Design review of the part built by this model. Coordinates are the model's own, in mm. A direction names the side the tool comes from. Round coordinates to 2 decimals unless told otherwise and drop trailing zeros. Order: outer loops, then holes, each group sorted by start corner. A loop starts at its lowest first (then second) coordinate and runs counter-clockwise, first axis right, second up.
Autodesk Inventor part; units mm, degrees
ref_plane "YZ Plane" through (0, 0, 0) normal (1, 0, 0) x (0, 1, 0)
ref_plane "XZ Plane" through (0, 0, 0) normal (0, 1, 0) x (-1, 0, 0)
ref_plane "XY Plane" through (0, 0, 0) normal (0, 0, 1) x (1, 0, 0)
sketch "Sketch1" plane through (0, 0, 0) normal (0, 1, 0) x (-1, 0, 0)
  line L0 (41.5, -27) -> (-41.5, -27)
  line L1 (-41.5, -27) -> (-41.5, 27)
  line L2 (-41.5, 27) -> (41.5, 27)
  line L3 (41.5, 27) -> (41.5, -27)
  line L4 (41.5, -27) -> (-41.5, 27) construction
  line L5 (-41.5, -27) -> (41.5, 27) construction
  point P0 (0, 0)
  dimension "d0" = 83
  dimension "d1" = 54
extrude "Extrusion1" add sketch "Sketch1" along normal blind 9
sketch "Sketch2" plane through (41.5, 0, 27) normal (1, 0, 0) x (0, 0, -1)
  line L0 (27, 0) -> (27, 8.8182) construction
  line L1 (27, 4.4091) -> (44.5, 4.4091) construction
  line L2 (44.5, 4.4091) -> (44.75, 4.4091)
  line L3 (44.75, 4.4091) -> (44.75, 11.998)
  line L4 (44.75, 11.998) -> (44.5, 11.998)
  line L5 (44.5, 11.998) -> (44.5, 4.4091)
  line L6 (9.5, 4.4091) -> (9.25, 4.4091)
  line L7 (9.25, 4.4091) -> (9.25, 11.998)
  line L8 (9.25, 11.998) -> (9.5, 11.998)
  line L9 (9.5, 11.998) -> (9.5, 4.4091)
  line L10 (26, 12.3352) -> (28, 12.3352)
  line L11 (28, 12.3352) -> (28, 5.3012)
  line L12 (28, 5.3012) -> (26, 5.3012)
  line L13 (26, 5.3012) -> (26, 12.3352)
  line L14 (26, 12.3352) -> (28, 5.3012) construction
  line L15 (28, 12.3352) -> (26, 5.3012) construction
  dimension "d4" = 17.5
  dimension "d5" = 0.25
  dimension "d6" = 2
  dimension "d7" = 7.034
extrude "Extrusion2" cut sketch "Sketch2" against normal blind 109.0125
properties part number "Small Bread Board" material "PC/ABS Plastic"
1) Take a section at A-A on y = 8. Give the boundary of the cut face in (x, z), plus the area to 3 significant figures.
Results:
outline: (-41.5, -27) - (41.5, -27) - (41.5, -17.75) - (-41.5, -17.75) - close; (-41.5, -17.5) - (41.5, -17.5) - (41.5, -1) - (-41.5, -1) - close; (-41.5, 1) - (41.5, 1) - (41.5, 17.5) - (-41.5, 17.5) - close; (-41.5, 17.75) - (41.5, 17.75) - (41.5, 27) - (-41.5, 27) - close
area: 4,270 mm2
2) Clearance check with a flat-ended pin moving along its axis: P1, Ø0.6, axis at x = -19.5, z = 0.5, coming from the +Y side. State where the tip first meets the part, or that it passes through.
Results:
P1: stops at y = 5.3
3) Take a section at B-B on x = 10. Give the boundary of the cut face in (y, z).
Results:
outline: (0, -27) - (9, -27) - (9, -17.75) - (4.41, -17.75) - (4.41, -17.5) - (9, -17.5) - (9, -1) - (5.3, -1) - (5.3, 1) - (9, 1) - (9, 17.5) - (4.41, 17.5) - (4.41, 17.75) - (9, 17.75) - (9, 27) - (0, 27) - close
4) For faces 1 (the face through (1, 4, 27)), 2 (the face through (1, 7, -17.75)), list the 3-axis set-ups (+Z, -Z, +X, -X, +Y, -Y) from which the entire face can be reached by the end or side of a thin tool; tool diameter is ignored.
Results:
face 1: +Z, +X, -X, +Y, -Y
face 2: +X, -X, +Y
5) To check wall thickness, follow line 1 along Z through (x, y) = (-36.5, 8.75); line 2 along Y through (x, z) = (-38, 0). State the ranges of each line that lie inside material, in increasing order.
Results:
line 1: z = -27 to -17.75, -17.5 to -1, 1 to 17.5, 17.75 to 27
line 2: y = 0 to 5.3
6) The part is to be moulded in two halves that separate along Z. For faces 3 (the face through (1, 7, 1)), 4 (the face through (1, 9, -9)), 5 (the face through (-1, 4, -27)), say which applies: released by +Z, released by -Z, zero draft, split by the parting line, or undercut.
Results:
face 3: undercut
face 4: zero draft
face 5: released by -Z
